Could you check a few things on this model? Use its own coordinates, in mm. Round coordinates to 2 decimals unless told otherwise and drop trailing zeros. Order: outer loops, then holes, each group sorted by start corner. A loop starts at its lowest first (then second) coordinate and runs counter-clockwise, first axis right, second up.
Autodesk Inventor part; units mm, degrees
ref_plane "YZ Plane" through (0, 0, 0) normal (1, 0, 0) x (0, 1, 0)
ref_plane "XZ Plane" through (0, 0, 0) normal (0, 1, 0) x (-1, 0, 0)
ref_plane "XY Plane" through (0, 0, 0) normal (0, 0, 1) x (1, 0, 0)
sketch "草图1" plane through (0, 0, 0) normal (0, 1, 0) x (-1, 0, 0)
  line L0 (-95, 54) -> (-66, 54)
  line L1 (-66, 54) -> (-66, 100)
  line L2 (-66, 100) -> (-95, 100)
  line L3 (-95, 100) -> (-95, 54)
  line L4 (-32, 144) -> (-32, 87)
  line L5 (-125, 0) -> (-125, 245)
  line L6 (-32, 87) -> (25, 87)
  line L7 (-125, 245) -> (-125, -245)
  line L8 (125, -245) -> (125, 245)
  line L9 (25, 144) -> (-32, 144)
  line L10 (-125, 245) -> (0, 245)
  line L11 (125, 245) -> (-125, 245)
  line L12 (25, 67) -> (-32, 67)
  line L13 (0, 0) -> (125, 0)
  line L14 (-32, 67) -> (-32, 10)
  line L15 (-32, 10) -> (25, 10)
  line L16 (3.5058, 0) -> (-3.4421, 0)
  line L17 (-66, -100) -> (-66, -54)
  line L18 (-95, -54) -> (-95, -100)
  line L19 (-95, -100) -> (-66, -100)
  line L20 (25, 87) -> (25, 144)
  line L21 (0, 245) -> (0, 0)
  line L22 (0, 245) -> (0, 0)
  line L23 (125, 0) -> (125, 245)
  line L24 (100, 15) -> (70, 15)
  line L25 (100, -15) -> (100, 15)
  line L26 (70, 15) -> (70, -15)
  line L27 (25, 10) -> (25, 67)
  line L28 (-125, -245) -> (125, -245)
  line L29 (-32, -87) -> (-32, -144)
  line L30 (-32, -10) -> (-32, -67)
  line L31 (25, -87) -> (-32, -87)
  line L32 (-32, -67) -> (25, -67)
  line L33 (25, -10) -> (-32, -10)
  line L34 (-32, -144) -> (25, -144)
  line L35 (-125, 0) -> (-125, -245)
  line L36 (25, -144) -> (25, -87)
  line L37 (25, -67) -> (25, -10)
  circle A0 centre (65, -182) radius 10
  line L38 (70, -15) -> (100, -15)
  line L39 (0, 0) -> (125, 0)
  line L40 (0, -245) -> (0, 0)
  line L41 (0, -245) -> (0, 0)
  line L42 (125, -245) -> (0, -245)
  line L43 (125, 0) -> (125, -245)
  line L44 (-125, -245) -> (0, -245)
  line L45 (0, 3) -> (0, -5)
  line L46 (-66, -54) -> (-95, -54)
  line L47 (0, 0) -> (-125, 0)
  line L48 (0, 0) -> (-125, 0)
  circle A1 centre (57.5, 194.9904) radius 1.5
  circle A2 centre (57.5, 169.0096) radius 1.5
  circle A3 centre (65, 182) radius 10
  circle A4 centre (65, 182) radius 15
  circle A5 centre (80, 182) radius 1.5
  line L49 (125, 245) -> (0, 245)
  circle A6 centre (65, -182) radius 15
  circle A7 centre (80, -182) radius 1.5
  circle A8 centre (57.5, -169.0096) radius 1.5
  circle A9 centre (57.5, -194.9904) radius 1.5
  point P0 (0, 144)
  point P1 (0, 10)
  point P2 (0, 67)
  point P3 (0, 87)
  dimension "d35" = 30
  dimension "d38" = 30
  dimension "d4" = 490
  dimension "d5" = 250
  dimension "d6" = 57
  dimension "d7" = 57
  dimension "d8" = 57
  dimension "d9" = 57
  dimension "d10" = 57
  dimension "d11" = 57
  dimension "d12" = 57
  dimension "d13" = 57
  dimension "d14" = 101
  dimension "d15" = 20
  dimension "d16" = 20
  dimension "d17" = 20
  dimension "d18" = 93
  dimension "d19" = 29
  dimension "d20" = 46
  dimension "d21" = 46
  dimension "d22" = 145
  dimension "d23" = 108
  dimension "d24" = 30
  dimension "d25" = 30
  dimension "d26" = 30
  dimension "d27" = 25
  dimension "d28" = 230
  dimension "d29" = 20
  dimension "d30" = 63
  dimension "d31" = 60
  dimension "d32" = 20
  dimension "d33" = 63
  dimension "d34" = 60
  dimension "d36" = 3
  dimension "d37" = 360
  dimension "d39" = 3
  dimension "d40" = 360
extrude "拉伸1" add sketch "草图1" along normal blind 10 contours L4 L6 L21 L12 L14 L15 L16 L47 L5 L10 L9
sketch "草图2" plane through (0, 0, 0) normal (0, -1, 0) x (1, 0, 0)
  line L0 (125, 0) -> (0, 0)
  line L1 (47, 159) -> (0, 159)
  line L2 (0, 159) -> (0, 0)
  line L3 (0, 0) -> (47, 0)
  line L4 (47, 0) -> (47, 159)
  line L5 (32, 10) -> (32, 67)
  line L6 (32, 144) -> (0, 144)
  line L7 (110, 115) -> (47, 115)
  line L8 (47, 115) -> (47, 39)
  line L9 (47, 39) -> (110, 39)
  line L10 (110, 39) -> (110, 115)
  line L11 (95, 54) -> (95, 100)
  line L12 (66, 100) -> (66, 54)
  line L13 (95, 100) -> (66, 100)
  line L14 (66, 54) -> (95, 54)
  dimension "d43" = 15
  dimension "d44" = 15
  dimension "d45" = 15
  dimension "d46" = 19
  dimension "d47" = 15
  dimension "d48" = 15
extrude "拉伸2" cut sketch "草图2" against normal blind 5
sketch "草图3" plane through (0, 10, 0) normal (0, 1, 0) x (1, 0, 0)
  line L0 (0, -159) -> (47, -159)
  line L1 (0, -245) -> (125, -245)
  line L2 (0, -159) -> (8, -159)
  line L3 (8, -159) -> (8, -245)
  line L4 (8, -245) -> (0, -245)
  line L5 (0, -245) -> (0, -159)
  point P0 (0, 0)
  dimension "d51" = 8
extrude "拉伸3" cut sketch "草图3" against normal blind 5
sketch "草图4" plane through (0, 5, 0) normal (0, 1, 0) x (1, 0, 0)
  circle A0 centre (4, -225) radius 2
  circle A1 centre (4, -179) radius 2
  line L0 (8, -159) -> (8, -245)
  line L1 (8, -245) -> (0, -245)
  line L2 (0, -159) -> (8, -159)
  point P0 (0, 0)
  dimension "d54" = 4
  dimension "d56" = 4
  dimension "d58" = 4
  dimension "d59" = 4
  dimension "d60" = 20
  dimension "d65" = 20
extrude "拉伸4" cut sketch "草图4" against normal blind 5
properties part number "top_3"
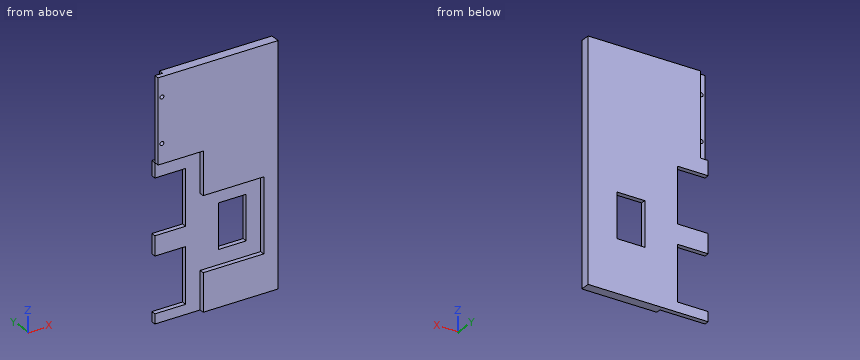
Q1. I need wall thicknesses on L1, parallel to Z at x = 4, y = 2.7; L2, parallel to X at y = 3.2, z = 225; L3, parallel to Z at x = 86, y = 2.5. Which ranges of each line are inside material? Lowest first, please.
Q2. Imagine slicing it at A-A, the plane y = 7.5. Please give me the cut outline in (x, z), then the cut area to 3 significant figures.
Q3. For P1, Ø1.5, axis at y = 2, z = 20.5, coming from the -X side; P2, Ø6.5, axis at x = 4, z = 225, coming from the +Y side; P3, Ø1.5, axis at x = 95.5, z = 65, coming from the -Y side, each with a flat end and sliding along its axis, tell me the tip position at first contact or that it passes through.
Q4. Imagine slicing it at D-D, the plane x = 76. Please give me the cut outline in (y, z).
Q5. Imagine slicing it at B-B, the plane x = 19.5. Please give me the cut outline in (y, z).
Q6. Imagine slicing it at C-C, the plane z = 96. Please give me the cut outline in (x, y), then the cut area to 3 significant figures.
Filled in:
1. L1: z = 159 to 177, 181 to 223, 227 to 245
1. L2: x = 0 to 2, 6 to 125
1. L3: z = 0 to 39, 115 to 245
2. outline: (0, 0) - (125, 0) - (125, 245) - (8, 245) - (8, 159) - (0, 159) - (0, 144) - (32, 144) - (32, 87) - (0, 87) - (0, 67) - (32, 67) - (32, 10) - (0, 10) - close; hole (66, 54) - (95, 54) - (95, 100) - (66, 100) - close
2. area: 25,000 mm2
3. P1: stops at x = 47
3. P2: stops at y = 5
3. P3: stops at y = 5
4. outline: (0, 0) - (10, 0) - (10, 54) - (5, 54) - (5, 39) - (0, 39) - close; (0, 115) - (5, 115) - (5, 100) - (10, 100) - (10, 245) - (0, 245) - close
5. outline: (0, 159) - (5, 159) - (5, 144) - (10, 144) - (10, 245) - (0, 245) - close; (5, 0) - (10, 0) - (10, 10) - (5, 10) - close; (5, 67) - (10, 67) - (10, 87) - (5, 87) - close
6. outline: (32, 5) - (66, 5) - (66, 10) - (32, 10) - close; (95, 5) - (110, 5) - (110, 0) - (125, 0) - (125, 10) - (95, 10) - close
6. area: 395 mm2
